```python
from build123d import *

# Parameters (mm, degrees)
BOSS_EXTRUDE1_DEPTH = 2
BOSS_EXTRUDE2_DEPTH = 2
SKETCH3_R           = 2
BOSS_EXTRUDE3_DEPTH = 2
BOSS_EXTRUDE4_DEPTH = 2
BOSS_EXTRUDE5_DEPTH = 4
CUT_EXTRUDE1_DEPTH  = 1


with BuildPart() as part:
    # Sketch1 → Boss-Extrude1 (new body)
    with BuildSketch(Plane.XY):
        with BuildLine():
            Line((-3, 0), (-6, 0))
            Line((-6, 0), (-6, -8))
            Line((-6, -8), (3, -8))
            Line((3, -8), (3, 0))
            Line((3, 0), (0, 0))
            Line((0, 0), (0, -1))
            ThreePointArc((0, -1), (-1.5, -2.5), (-3, -1))
            Line((-3, -1), (-3, 0))
        make_face()
    extrude(amount=BOSS_EXTRUDE1_DEPTH)

    # Sketch2 → Boss-Extrude2 (add)
    with BuildSketch(Plane(origin=(3, 0, 0), x_dir=(0, 0, -1), z_dir=(1, 0, 0))):
        with BuildLine():
            Line((0, 0), (3, 0))
            Line((3, 0), (3, -2.002573702))
            ThreePointArc((3, -2.002573702), (1.071733869, -4.001286851), (3, -6))
            Line((3, -6), (3, -8))
            Line((3, -8), (0, -8))
            Line((0, -8), (0, 0))
        make_face()
    extrude(amount=-BOSS_EXTRUDE2_DEPTH)

    # Sketch3 → Boss-Extrude3 (add)
    with BuildSketch(Plane.ZY.offset(6)):
        with BuildLine():
            Line((-3, 0), (0, 0))
            Line((0, 0), (0, -8))
            Line((0, -8), (-3, -8))
            ThreePointArc((-3, -8), (-7, -4), (-3, 0))
        make_face()
        with Locations((-3, -4)):
            Circle(SKETCH3_R, mode=Mode.SUBTRACT)
    extrude(amount=-BOSS_EXTRUDE3_DEPTH)

    # Sketch4 → Boss-Extrude4 (add)
    with BuildSketch(Plane.ZY.offset(6)):
        with BuildLine():
            Line((6, -8), (2, -8))
            Line((2, -8), (2, 0))
            Line((2, 0), (6, -2.994386604))
            Line((6, -2.994386604), (6, -3.994386604))
            Line((6, -3.994386604), (5, -3.994386604))
            ThreePointArc((5, -3.994386604), (3.997193302, -4.997193302), (5, -6))
            Line((5, -6), (6, -6))
            Line((6, -6), (6, -8))
        make_face()
    extrude(amount=-BOSS_EXTRUDE4_DEPTH)

    # Sketch5 → Boss-Extrude5 (add)
    with BuildSketch(Plane.XZ.offset(8)):
        with BuildLine():
            Line((3, 2), (1, 2))
            ThreePointArc((1, 2), (0.414213562, 3.414213562), (-1, 4))
            Line((-1, 4), (-1, 6))
            ThreePointArc((-1, 6), (1.828427125, 4.828427125), (3, 2))
        make_face()
    extrude(amount=-BOSS_EXTRUDE5_DEPTH)

    # Sketch6 → Cut-Extrude1 (cut)
    with BuildSketch(Plane.XZ.offset(8)):
        with BuildLine():
            Line((-0.007843258, 5.875), (2.872983346, 3))
            ThreePointArc((2.872983346, 3), (1.825562469, 4.831288882), (-0.007843258, 5.875))
        make_face()
    extrude(amount=-CUT_EXTRUDE1_DEPTH, mode=Mode.SUBTRACT)


solid = part.part
```
Can you work these out from the model? Positions are in its coordinate system, mm. A direction names the side the tool comes from. Give positions to 0.01 mm unless a question says otherwise; leave off trailing zeros. Order: outer loops, then holes, each group sorted by start corner. A loop starts at its lowest first (then second) coordinate and runs counter-clockwise, first axis right, second up. Notation, with made-up numbers: M 41,76 L 59,76 A3 ccw 59,81 Z; hole C 20,-2 d5. An arc over 180 degrees is marked long. One line per item, written item: value.
1) Please list where these lines run through material, in increasing order: line 1 along Y through (x, z) = (-5.25, -3); line 2 along X through (y, z) = (-6.5, -0.5); line 3 along Z through (x, y) = (-3, -6).
Answer sheet:
line 1: y = -8 to -6, -2 to 0
line 2: x = -6 to -4, 1 to 3
line 3: z = 0 to 2
2) For P1, Ø2, axis at x = 1.5, y = -7, coming from the -Z side; P2, Ø0.5, axis at x = -5, z = 5.5, coming from the +Y side; P3, Ø1, axis at x = -1.5, y = -3.5, coming from the +Z side, each with a flat end and sliding along its axis, tell me the tip position at first contact or that it passes through.
Answer sheet:
P1: stops at z = -3
P2: stops at y = -2.43
P3: stops at z = 2
3) We'd pull the mould along Y, two halves only. Please class faces 4 (the face through (-1.4, -8, 1.6)), 5 (the face through (-5, -6, 5.5)), 6 (the face through (2, 0, 0)), 7 (the face through (1, -3.9, -0.9)): released by +Y, released by -Y, zero draft, split by the parting line, or undercut.
Answer sheet:
face 4: released by -Y
face 5: undercut
face 6: released by +Y
face 7: zero draft
4) I want a section at B-B, the plane y = -3.5. List the corners of the cut face in (x, z) for me.
Answer sheet:
outline: M -6,-6.97 L -4,-6.97 L -4,-4.94 L -6,-4.94 Z; M -6,-1.06 L -4,-1.06 L -4,0 L 1,0 L 1,-1.14 L 3,-1.14 L 3,2 L -4,2 L -4,6 L -6,6 Z
5) I want a section at D-D, the plane x = -1.5. List the corners of the cut face in (y, z) for me.
Answer sheet:
outline: M -8,0 L -2.5,0 L -2.5,2 L -8,2 Z
6) I want a section at A-A, the plane z = -1.75. List the corners of the cut face in (x, y) for me, plus the area to 3 significant figures.
Answer sheet:
outline: M -6,-8 L -4,-8 L -4,-5.56 L -6,-5.56 Z; M -6,-2.44 L -4,-2.44 L -4,0 L -6,0 Z; M 1,-8 L 3,-8 L 3,-5.5 L 1,-5.5 Z; M 1,-2.5 L 3,-2.5 L 3,0 L 1,0 Z
area: 19.8 mm^2
7) On a 3-axis mill with a long thin cutter (end or side, diameter ignored), from which of +Z, -Z, +X, -X, +Y, -Y can I reach the whole of each face in a straight line? I mean faces 1 (the face through (1, -4, 4)), 2 (the face through (0.43, -6.03, 3.4)), 3 (the face through (2, -7, -3)). Say none if no direction works.
Answer sheet:
face 1: +Z, +X, +Y
face 2: +Y, -Y
face 3: -Z, +X, +Y, -Y
8) I want a section at C-C, the plane z = 1.5. List the corners of the cut face in (x, y) for me.
Answer sheet:
outline: M -6,-8 L 3,-8 L 3,0 L 0,0 L 0,-1 A1.5 cw -3,-1 L -3,0 L -6,0 Z
